Geometry: see drawing. Coordinates: mm, zero at the bounding-box minimum. A direction names the side the tool comes from. Coordinates: 2 decimals unless noted, no trailing zeros. Loops run counter-clockwise (first coordinate to the right, second up) from the corner with the lowest first, then second, coordinate; pieces in that order, holes last. Notation, with made-up numbers: (17, -15.5) - (35, -15.5) arc R24 cw to (35, 13.5) - close; hole circle Ø10 at (51.5, 22). An arc over 180 degrees is marked (long way). Use a Markdown table: item, result. Add a question column.
1. Section query D-D on z = 5. Return the cut outline in (x, y).
2. Section query C-C on z = 19.75. Return the cut outline in (x, y), then the cut area to 3 significant figures.
3. Access query for the marked faces 1, 2 and 3. Directions: +Z, -Z, +X, -X, +Y, -Y. A direction counts if a zero-diameter tool reaches every point of the face in a straight line with its end or side. Return the directions, or none.
4. Draft query along Z for the marked faces 4, 5, 6 and 7. Return one class per face: released by +Z, released by -Z, zero draft, split by the parting line, or undercut.
5. Contact query for flat-ended pins moving along their axis: P1, Ø2.5, axis at y = 18, z = 5.5, coming from the -X side; P2, Ø4, axis at x = 10.5, z = 19, coming from the +Y side; P3, Ø2.5, axis at x = 10, z = 18, coming from the -Y side; P4, Ø6, axis at x = 13.5, z = 11.5, coming from the -Y side. Output: stop coordinate, or through.
6. Ray query, L1, parallel to X at y = 13.6, z = 18; L2, parallel to X at y = 19, z = 8.5; L3, parallel to Y at x = 16.25, z = 11.5. Return the intervals inside material, ascending. Write a range as [from, to].
7. Section query A-A on y = 12.5. Return the cut outline in (x, z), then the cut area to 3 significant figures.
8. Section query B-B on x = 10. Return the cut outline in (y, z).
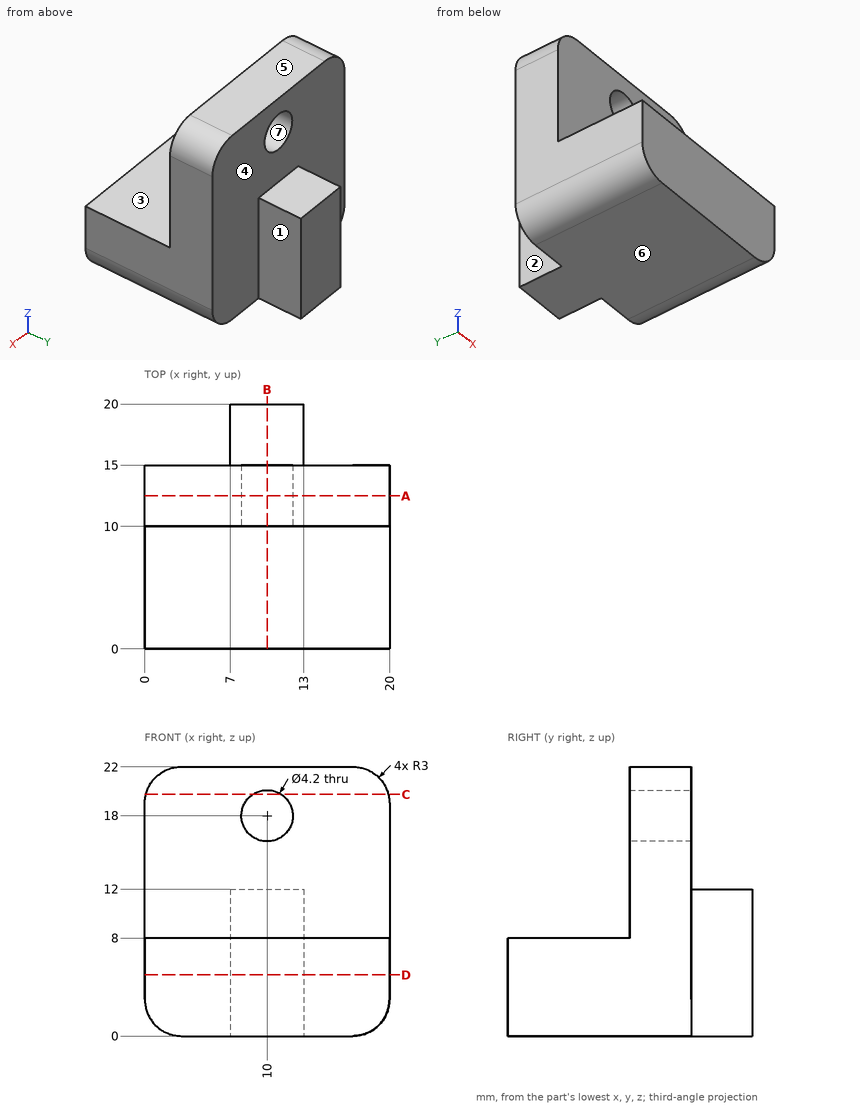
Resolved:
| question | item | result |
|---|---|---|
| 1 | outline | (0, 0) - (20, 0) - (20, 15) - (13, 15) - (13, 20) - (7, 20) - (7, 15) - (0, 15) - close |
| 2 | outline | (0.1, 10) - (8.84, 10) - (8.84, 15) - (0.1, 15) - close; (11.16, 10) - (19.9, 10) - (19.9, 15) - (11.16, 15) - close |
| 2 | area | 87.4 mm² |
| 3 | face 1 | +Z, -Z, +X, +Y |
| 3 | face 2 | +Z, -Z, -X, +Y |
| 3 | face 3 | +Z, +X, -X, -Y |
| 4 | face 4 | zero draft |
| 4 | face 5 | released by +Z |
| 4 | face 6 | released by -Z |
| 4 | face 7 | undercut |
| 5 | P1 | x = 7 |
| 5 | P2 | y = 15 |
| 5 | P3 | through |
| 5 | P4 | y = 10 |
| 6 | L1 | [0, 7.9], [12.1, 20] |
| 6 | L2 | [7, 13] |
| 6 | L3 | [10, 15] |
| 7 | outline | (0, 3) arc R3 ccw to (3, 0) - (17, 0) arc R3 ccw to (20, 3) - (20, 19) arc R3 ccw to (17, 22) - (3, 22) arc R3 ccw to (0, 19) - close; hole circle Ø4.2 at (10, 18) |
| 7 | area | 418 mm² |
| 8 | outline | (0, 0) - (20, 0) - (20, 12) - (15, 12) - (15, 15.9) - (10, 15.9) - (10, 8) - (0, 8) - close; (10, 20.1) - (15, 20.1) - (15, 22) - (10, 22) - close |
